from build123d import *

# Parameters (mm, degrees)
BOSS_EXTRUDE1_DEPTH     = 57
SKETCH2_R               = 37.5
BOSS_EXTRUDE2_DEPTH     = 2
CUT_EXTRUDE2_DEPTH      = 186.90387301
CUT_EXTRUDE2_DEPTH_BACK = 186.90387301
SKETCH3_W               = 110
SKETCH3_H               = 54


with BuildPart() as part:
    # Sketch1 → Boss-Extrude1 (new, symmetric)
    with BuildSketch(Plane.XY):
        with BuildLine():
            Line((0, 50), (-165, 58.5))
            Line((-165, 58.5), (-165, -58.5))
            Line((-165, -58.5), (0, -50))
            ThreePointArc((0, -50), (50, 0), (0, 50))
        make_face()
    extrude(amount=BOSS_EXTRUDE1_DEPTH, both=True)

    # Sketch2 → Boss-Extrude2 (add)
    with BuildSketch(Plane.ZY.offset(165)):
        Circle(SKETCH2_R)
    extrude(amount=BOSS_EXTRUDE2_DEPTH)

    # Sketch3 → Cut-Extrude2 (cut, two sides: drawn at the far end of the back side and taken through both)
    with BuildSketch(Plane(origin=(0, 0, 0), x_dir=(1, 0, 0), z_dir=(0, 1, 0)).offset(-CUT_EXTRUDE2_DEPTH_BACK)):
        with Locations((-5, 0)):
            Rectangle(SKETCH3_W, SKETCH3_H)
    extrude(amount=CUT_EXTRUDE2_DEPTH + CUT_EXTRUDE2_DEPTH_BACK, mode=Mode.SUBTRACT)


solid = part.part
Geometry: final body of the model. Coordinates: model frame, mm. A direction names the side the tool comes from. Round coordinates to 2 decimals unless told otherwise and drop trailing zeros. Loops run counter-clockwise (first coordinate to the right, second up) from the corner with the lowest first, then second, coordinate; pieces in that order, holes last.
Q1. Section B-B on x = -34. Return loops of the section in (y, z), plus the area to 3 significant figures.
Q2. Material intervals for L1, parallel to Z at x = -52, y = 20; L2, parallel to X at y = -5, z = -3; L3, parallel to X at y = 0.5, z = -46, sorted ascending.
Q3. Section D-D on x = 26.5. Return loops of the section in (y, z), plus the area to 3 significant figures.
Q4. Access query for faces 4 (the flat face through (-101.988, -55.254, 0.798)), 5 (the flat face through (-6, -1, 27)), 6 (the flat face through (-165, 1, 39)). Directions: +Z, -Z, +X, -X, +Y, -Y. A direction counts if a zero-diameter tool reaches every point of the face in a straight line with its end or side. Return the directions, or none.
Q5. Pull-direction query (Z, two-part tool) for faces 1 (the flat face through (-99.678, 55.135, 0.798)), 2 (the flat face through (-6, -1, -27)), 3 (the flat face through (-59, 1, 57)); classes: released by +Z, released by -Z, zero draft, split by the parting line, or undercut.
Q6. Pin query (flat end, axial travel): P1, Ø10, axis at y = -31.5, z = 36.5, coming from the +X side; P2, Ø8, axis at y = 25.5, z = 35, coming from the -X side; P3, Ø4, axis at x = -133.5, z = -20, coming from the -Y side. Return the tip coordinate at first contact, or that it passes through.
Q7. Section C-C on z = 0. Return loops of the section in (x, y).
Q8. Section A-A on y = 0. Return loops of the section in (x, z).
Evaluation:
1. outline: (-51.75, -57) - (51.75, -57) - (51.75, -27) - (-51.75, -27) - close; (-51.75, 27) - (51.75, 27) - (51.75, 57) - (-51.75, 57) - close
1. area: 6,210 mm2
2. L1: z = -57 to -27, 27 to 57
2. L2: x = -167 to -60
2. L3: x = -165 to 50
3. outline: (-42.4, -57) - (42.4, -57) - (42.4, -27) - (-42.4, -27) - close; (-42.4, 27) - (42.4, 27) - (42.4, 57) - (-42.4, 57) - close
3. area: 5,090 mm2
4. face 4: +Z, -Z, +X, -Y
4. face 5: +X, +Y, -Y
4. face 6: -X
5. face 1: zero draft
5. face 2: undercut
5. face 3: released by +Z
6. P1: stops at x = 42.4
6. P2: stops at x = -165
6. P3: stops at y = -56.98
7. outline: (-167, -37.5) - (-165, -37.5) - (-165, -58.5) - (-60, -53.09) - (-60, 53.09) - (-165, 58.5) - (-165, 37.5) - (-167, 37.5) - close
8. outline: (-167, -37.5) - (-165, -37.5) - (-165, -57) - (50, -57) - (50, -27) - (-60, -27) - (-60, 27) - (50, 27) - (50, 57) - (-165, 57) - (-165, 37.5) - (-167, 37.5) - close
